from build123d import *

# Parameters (mm, degrees)
F1_DEPTH = 61
F0_R     = 9
F2_DEPTH = 15
F4_DEPTH = 30


with BuildPart() as f1:
    # F0 (on Top) → F1 (new body)
    with BuildSketch(Plane.XY):
        Polygon((0, 15.107143), (-27.166667, 15.107143), (-27.166667, -20.892857), (-27.166667, -45.892857), (-15, -45.892857), (-15, 11.464287), (0, 11.464287), (15, 11.464287), (15, -45.892857), (27.166667, -45.892857), (27.166667, -20.892857), (27.166667, 15.107143), align=None)
    extrude(amount=F1_DEPTH)

    # F0 (on Top) → F2 (join)
    with BuildSketch(Plane.XY):
        with BuildLine():
            Line((-27.166667, 15.107143), (-96.696436, 15.107143))
            ThreePointArc((-96.696436, 15.107143), (-114.696436, -2.892857), (-96.696436, -20.892857))
            ThreePointArc((-96.696436, -20.892857), (-93.708552, -20.64314), (-90.803571, -19.900918))
            Line((-90.803571, -19.900918), (-90.803571, -20.892857))
            Line((-90.803571, -20.892857), (-27.166667, -20.892857))
            Line((-27.166667, -20.892857), (-27.166667, 15.107143))
        make_face()
        with Locations((-96.696436, -2.892857)):
            Circle(F0_R, mode=Mode.SUBTRACT)
        Polygon((0, 15.107143), (-27.166667, 15.107143), (-27.166667, -20.892857), (-27.166667, -45.892857), (-15, -45.892857), (-15, 11.464287), (0, 11.464287), (15, 11.464287), (15, -45.892857), (27.166667, -45.892857), (27.166667, -20.892857), (27.166667, 15.107143), align=None)
        with BuildLine():
            ThreePointArc((-90.803571, -19.900918), (-93.708552, -20.64314), (-96.696436, -20.892857))
            Line((-96.696436, -20.892857), (-90.803571, -20.892857))
            Line((-90.803571, -20.892857), (-90.803571, -19.900918))
        make_face()
        with BuildLine():
            Line((96.696436, 15.107143), (27.166667, 15.107143))
            Line((27.166667, 15.107143), (27.166667, -20.892857))
            Line((27.166667, -20.892857), (96.696436, -20.892857))
            ThreePointArc((96.696436, -20.892857), (114.696436, -2.892857), (96.696436, 15.107143))
        make_face()
        with Locations((96.696436, -2.892857)):
            Circle(F0_R, mode=Mode.SUBTRACT)
    extrude(amount=F2_DEPTH)

    # F3 (on face) → F4 (join)
    with BuildSketch(Plane(origin=(15, 0, 0), x_dir=(0, -1, 0), z_dir=(-1, 0, 0))):
        Polygon((45.892857, 0), (-11.464287, 61), (-11.464287, 0), align=None)
    extrude(amount=F4_DEPTH)


solid = f1.part
Read the model definition and answer for the solid it produces. Units are mm, in the model's axes. A direction names the side the tool comes from. Round coordinates to 2 decimals unless told otherwise and drop trailing zeros. Write each loop counter-clockwise with the first axis right and the second up, starting at its lowest first coordinate (ties: lowest second). Pieces come first, ordered by that corner, then holes. Notation, with made-up numbers: M -22.5,-6.5 L 12.5,-6.5 A3 ccw 12.5,-1.5 Z; hole C 6.25,61 d7. An arc over 180 degrees is marked long. Use a Markdown table: item, result.
1) The part is cut by section A-A (y = -7). Write down the section's boundary in (x, z), plus the area to 3 significant figures.
Answers follow:
| item | result |
|---|---|
| outline | M -114.22,0 L -104.7,0 L -104.7,15 L -114.22,15 Z; M -88.69,0 L 88.69,0 L 88.69,15 L 27.17,15 L 27.17,61 L 15,61 L 15,41.36 L -15,41.36 L -15,61 L -27.17,61 L -27.17,15 L -88.69,15 Z; M 104.7,0 L 114.22,0 L 114.22,15 L 104.7,15 Z |
| area | 4,860 mm2 |
2) The part is cut by section C-C (z = 30.5). Write down the section's boundary in (x, y).
Answers follow:
| item | result |
|---|---|
| outline | M -27.17,-45.89 L -15,-45.89 L -15,-17.21 L 15,-17.21 L 15,-45.89 L 27.17,-45.89 L 27.17,15.11 L -27.17,15.11 Z |
3) The part is cut by section B-B (z = 4). Write down the section's boundary in (x, y).
Answers follow:
| item | result |
|---|---|
| outline | M -96.7,-20.89 L -27.17,-20.89 L -27.17,-45.89 L -15,-45.89 L -15,-42.13 L 15,-42.13 L 15,-45.89 L 27.17,-45.89 L 27.17,-20.89 L 96.7,-20.89 A18 ccw 96.7,15.11 L -96.7,15.11 A18 ccw Z; hole C -96.7,-2.89 d18; hole C 96.7,-2.89 d18 |
4) The part is cut by section D-D (x = 43). Write down the section's boundary in (y, z), plus the area to 3 significant figures.
Answers follow:
| item | result |
|---|---|
| outline | M -20.89,0 L 15.11,0 L 15.11,15 L -20.89,15 Z |
| area | 540 mm2 |
5) Flat-ended cylindrical pins translate along their axes: pin 1 (12 mm diameter, centred on x = 63.5, z = 5.5, fed in from -Y); pin 2 (1 mm diameter, centred on y = -1, z = 19.5, fed in from +X); pin 3 (10 mm diameter, centred on x = 70.5, y = -1, fed in from +Z). Find the tip coordinate at first contact, or state that the pin passes through.
Answers follow:
| item | result |
|---|---|
| pin 1 | stops at y = -20.89 |
| pin 2 | stops at x = 27.17 |
| pin 3 | stops at z = 15 |
6) For a pull along Y with two mould halves and no side action, classify faces 1 (the flat face through (15, -30, 44)), 2 (the cylindrical face through (89.554, -8.369, 7.395)), 3 (the flat face through (1, 15.107, 23)) as pulls with the +Y half, pulls with the -Y half, needs draft (parallel to the pull), parting line crosses it, or undercut.
Answers follow:
| item | result |
|---|---|
| face 1 | needs draft |
| face 2 | undercut |
| face 3 | pulls with the +Y half |
7) Straight lines are drawn through the part: line 1 along X through (y, z) = (-24.5, 47.5); line 2 along X through (y, z) = (-0.5, 31.5); line 3 along Z through (x, y) = (52.5, 0.5). For each, find the intervals that lie inside material, in ascending order. Write a range as [from, to].
Answers follow:
| item | result |
|---|---|
| line 1 | x = [-27.17, -15], [15, 27.17] |
| line 2 | x = [-27.17, 27.17] |
| line 3 | z = [0, 15] |
8) A tool of negligible diameter and unlimited length cuts with its end or side. For faces 4 (the flat face through (-62, -20.893, 7)), 5 (the flat face through (-72, -3, 15)), 6 (the flat face through (-15, -30, 44)), 7 (the flat face through (70, -3, 15)), from which of +Z, -Z, +X, -X, +Y, -Y can it reach the whole face along a straight path? Write none if from no direction.
Answers follow:
| item | result |
|---|---|
| face 4 | +Z, -Z, -X, -Y |
| face 5 | +Z, -X, +Y, -Y |
| face 6 | +Z, -Y |
| face 7 | +Z, +X, +Y, -Y |
